from build123d import *

# Parameters (mm, degrees)
SKETCH1_R           = 36
SKETCH1_R_2         = 31.1
BOSS_EXTRUDE1_DEPTH = 15
SKETCH2_R           = 36
BOSS_EXTRUDE2_DEPTH = 5
SKETCH3_R           = 22.5
CUT_EXTRUDE1_DEPTH  = 5
SKETCH4_R           = 5
BOSS_EXTRUDE3_DEPTH = 20
BOSS_EXTRUDE4_DEPTH = 20
SKETCH7_R           = 2.25
CUT_EXTRUDE2_DEPTH  = 78.645922206
SKETCH9_W           = 8.35
SKETCH9_H           = 20
BOSS_EXTRUDE5_DEPTH = 10
FILLET1_R           = 12
SKETCH10_R          = 3
CUT_EXTRUDE3_DEPTH  = 30
CUT_EXTRUDE5_START  = -5
SKETCH10_4_R        = 5.5
SKETCH10_4_R_2      = 3
CUT_EXTRUDE5_DEPTH  = 25
FILLET2_R           = 3
FILLET3_R           = 1


with BuildPart() as part:
    # Sketch1 → Boss-Extrude1 (new body)
    with BuildSketch(Plane.XY):
        Circle(SKETCH1_R)
        Circle(SKETCH1_R_2, mode=Mode.SUBTRACT)
    extrude(amount=BOSS_EXTRUDE1_DEPTH)

    # Sketch2 → Boss-Extrude2 (add)
    with BuildSketch(Plane.XY.offset(15)):
        Circle(SKETCH2_R)
    extrude(amount=BOSS_EXTRUDE2_DEPTH)

    # Sketch3 → Cut-Extrude1 (cut)
    with BuildSketch(Plane.XY.offset(20)):
        Circle(SKETCH3_R)
    extrude(amount=-CUT_EXTRUDE1_DEPTH, mode=Mode.SUBTRACT)

    # Sketch4 → Boss-Extrude3 (add)
    with BuildSketch(Plane(origin=(0, 0, 0), x_dir=(-1, 0, 0), z_dir=(0, 0, -1))):
        with Locations((0, 36.1)):
            Circle(SKETCH4_R)
        with Locations((31.263517077, 18.05)):
            Circle(SKETCH4_R)
        with Locations((31.263517077, -18.05)):
            Circle(SKETCH4_R)
        with Locations((0, -36.1)):
            Circle(SKETCH4_R)
        with Locations((-31.263517077, -18.05)):
            Circle(SKETCH4_R)
        with Locations((-31.263517077, 18.05)):
            Circle(SKETCH4_R)
    extrude(amount=-BOSS_EXTRUDE3_DEPTH)

    # Sketch8 → Boss-Extrude4 (add)
    with BuildSketch(Plane(origin=(0, 0, 0), x_dir=(-1, 0, 0), z_dir=(0, 0, -1))):
        with BuildLine():
            Line((-28.387135314, -22.139795588), (-9.877135314, -54.200056036))
            Line((-9.877135314, -54.200056036), (51.877193071, -18.54617792))
            Line((51.877193071, -18.54617792), (33.367193071, 13.514082528))
            ThreePointArc((33.367193071, 13.514082528), (18, -31.176914536), (-28.387135314, -22.139795588))
        make_face()
    extrude(amount=-BOSS_EXTRUDE4_DEPTH)

    # Sketch7 → Cut-Extrude2 (cut, through all)
    with BuildSketch(Plane(origin=(0, 0, 0), x_dir=(-1, 0, 0), z_dir=(0, 0, -1))):
        with Locations((-31.263517077, 18.05)):
            Circle(SKETCH7_R)
        with Locations((0, 36.1)):
            Circle(SKETCH7_R)
        with Locations((31.263517077, 18.05)):
            Circle(SKETCH7_R)
        with Locations((31.263517077, -18.05)):
            Circle(SKETCH7_R)
        with Locations((0, -36.1)):
            Circle(SKETCH7_R)
        with Locations((-31.263517077, -18.05)):
            Circle(SKETCH7_R)
    extrude(amount=-CUT_EXTRUDE2_DEPTH, mode=Mode.SUBTRACT)

    # Sketch9 → Boss-Extrude5 (add)
    with BuildSketch(Plane(origin=(-21.000028879, -36.373116978, 0), x_dir=(0.8660254037844385, -0.5000000000000004, 0), z_dir=(-0.5000000000000003, -0.8660254037844384, 0))):
        with Locations((-39.828878116, 10)):
            Rectangle(SKETCH9_W, SKETCH9_H)
        with Locations((39.828878116, 10)):
            Rectangle(SKETCH9_W, SKETCH9_H)
    extrude(amount=-BOSS_EXTRUDE5_DEPTH)

    # Fillet1
    # the kernel refuses this fillet: 12 mm, written as the material it adds along each edge
    with BuildSketch(Plane(origin=(-46.877193071, -9.885923882, 20), x_dir=(-0.8660254037844379, 0.500000000000001, 0), z_dir=(0, 0, -1))) as fillet1_piece_1:
        with BuildLine():
            CenterArc((12, 11.431425983), FILLET1_R, 180, 72.29196439)
            Line((0, 11.431425983), (-0.24, 11.431425983))
            Line((-0.24, 11.431425983), (-0.24, 0))
            Line((-0.24, 0), (0, -0.24))
            ThreePointArc((0, -0.24), (4.175, -0.24), (8.277, -0.22862852))
            Line((8.277, -0.22862852), (8.35, 0))
        make_face()
    extrude(amount=20)
    with BuildSketch(Plane(origin=(14.877135314, -45.539801998, 20), x_dir=(0.5000000000000003, 0.8660254037844385, 0), z_dir=(0, 0, -1))) as fillet1_piece_2:
        with BuildLine():
            CenterArc((11.431425983, 12), FILLET1_R, 197.70803561, 72.29196439)
            Line((0, 8.35), (-0.22862852, 8.277))
            ThreePointArc((-0.22862852, 8.277), (-0.24, 4.175), (-0.24, 0))
            Line((-0.24, 0), (0, -0.24))
            Line((0, -0.24), (11.431425983, -0.24))
            Line((11.431425983, -0.24), (11.431425983, 0))
        make_face()
    extrude(amount=20)

    # Sketch10 → Cut-Extrude3 (cut)
    with BuildSketch(Plane(origin=(-21.000028879, -36.373116978, 0), x_dir=(0.8660254037844385, -0.5000000000000004, 0), z_dir=(-0.5000000000000003, -0.8660254037844384, 0))):
        with Locations((37.503878116, 10)):
            Circle(SKETCH10_R)
        with Locations((-37.503878116, 10)):
            Circle(SKETCH10_R)
    extrude(amount=-CUT_EXTRUDE3_DEPTH, mode=Mode.SUBTRACT)

    # Sketch10<4> → Cut-Extrude5 (cut)
    # profile 1 of 2: a face of its own
    with BuildSketch(Plane(origin=(-21.000028879, -36.373116978, 0), x_dir=(0.8660254037844385, -0.5000000000000004, 0), z_dir=(-0.5000000000000003, -0.8660254037844384, 0)).offset(CUT_EXTRUDE5_START)):
        with Locations((37.503878116, 10)):
            Circle(SKETCH10_4_R)
        with Locations((37.503878116, 10)):
            Circle(SKETCH10_4_R_2, mode=Mode.SUBTRACT)
    # profile 2 of 2: a face of its own
    with BuildSketch(Plane(origin=(-21.000028879, -36.373116978, 0), x_dir=(0.8660254037844385, -0.5000000000000004, 0), z_dir=(-0.5000000000000003, -0.8660254037844384, 0)).offset(CUT_EXTRUDE5_START)):
        with Locations(Location((-37.503878116, 10, 0), (0, 0, 289.655481315))):
            Circle(SKETCH10_4_R)
        with Locations((-37.503878116, 10)):
            Circle(SKETCH10_4_R_2, mode=Mode.SUBTRACT)
    extrude(amount=-CUT_EXTRUDE5_DEPTH, mode=Mode.SUBTRACT)

    # Fillet2
    fillet2_edges = [part.edges().sort_by_distance(p)[0] for p in [
        (-56.608505192, -10.041050901, 0),
        (-56.608505192, -10.041050901, 20),
        (19.608447435, -54.044929017, 0),
        (19.608447435, -54.044929017, 20),
    ]]
    fillet(fillet2_edges, radius=FILLET2_R)

    # Fillet3
    fillet3_edges = [part.edges().sort_by_distance(p)[0] for p in [
        (-52.581487065, -12.366050901, 15.179527005),
        (9.21614259, -48.044929017, 10),
    ]]
    fillet(fillet3_edges, radius=FILLET3_R)


solid = part.part
Could you check a few things on this model? Use its own coordinates, in mm. A direction names the side the tool comes from. Coordinates: 2 decimals unless noted, no trailing zeros. Loops run counter-clockwise (first coordinate to the right, second up) from the corner with the lowest first, then second, coordinate; pieces in that order, holes last.
1. Imagine slicing it at C-C (z = 1.5). Please give me the cut outline in (x, y).
2. Imagine slicing it at D-D (x = -19.5). Please give me the cut outline in (y, z), and give its area (3 significant figures).
3. We'd pull the mould along Y, two halves only. Please class faces 4 (the face through (-56.644, -10.102, 9.902)), 5 (the face through (19.57, -54.11, 9.9)), 6 (the face through (0.29, 38.33, 9.86)): released by +Y, released by -Y, zero draft, split by the parting line, or undercut.
4. For faces 1 (the face through (-36.453, 8.17, 9.86)), 2 (the face through (-35.55, 6.67, 10.62)), 3 (the face through (19.23, -52.9, 0.86)), which set-ups out of +Z, -Z, +X, -X, +Y, -Y let a thin tool reach every point of the face, with its end or its side?
5. Imagine slicing it at A-A (x = 0). Please give me the cut outline in (y, z).
6. Imagine slicing it at B-B (y = 9). Please give me the cut outline in (x, z), and give its area (3 significant figures).
7. I need wall thicknesses on L1, parallel to Y at x = 10.5, z = 13; L2, parallel to Y at x = 0, z = 6.75; L3, parallel to Y at x = 21.5, z = 7.75. Which ranges of each line are inside material? Lowest first, please.
8. For P1, Ø7, axis at x = 31.26, y = 18.05, coming from the -Z side; P2, Ø12, axis at x = -13.5, z = 3.5, coming from the +Y side; P3, Ø4, axis at x = 26, z = 5.5, coming from the -Y side; P4, Ø2, axis at x = -31, z = 4.5, coming from the -Y side, each with a flat end and sliding along its axis, tell me the tip position at first contact or that it passes through.
Computed values:
1. outline: (-58.76, -14.57) - (16.76, -58.17) - (21.83, -49.4) arc R12 cw to (20.59, -35.64) - (28.39, -22.14) arc R5 ccw (long way) to (33.37, -13.51) arc R36 ccw to (33.37, 13.51) arc R5 ccw (long way) to (28.39, 22.14) arc R36 ccw to (4.98, 35.65) arc R5 ccw (long way) to (-4.98, 35.65) arc R36 ccw to (-28.39, 22.14) arc R5 ccw (long way) to (-33.37, 13.51) - (-41.16, 0.01) arc R12 cw to (-53.69, -5.79) - close; hole circle Ø4.5 at (-31.26, -18.05); hole circle Ø4.5 at (-31.26, 18.05); hole circle Ø62.2 at (0, 0); hole circle Ø4.5 at (0, -36.1); hole circle Ø4.5 at (0, 36.1); hole circle Ø4.5 at (31.26, -18.05); hole circle Ø4.5 at (31.26, 18.05)
2. outline: (-37.24, 0) - (-24.23, 0) - (-24.23, 15) - (-11.22, 15) - (-11.22, 20) - (-37.24, 20) - close; (11.22, 15) - (24.23, 15) - (24.23, 0) - (30.26, 0) - (30.26, 20) - (11.22, 20) - close
2. area: 511 mm2
3. face 4: released by +Y
3. face 5: released by -Y
3. face 6: undercut
4. face 1: +Z, -Z, -X
4. face 2: -X
4. face 3: -Z, +X, -Y
5. outline: (-48.5, 0) - (-38.35, 0) - (-38.35, 20) - (-48.5, 20) - close; (-33.85, 0) - (-31.1, 0) - (-31.1, 15) - (-22.5, 15) - (-22.5, 20) - (-33.85, 20) - close; (22.5, 15) - (31.1, 15) - (31.1, 0) - (33.85, 0) - (33.85, 20) - (22.5, 20) - close; (38.35, 0) - (41.1, 0) - (41.1, 20) - (38.35, 20) - close
6. outline: (-35.97, 0) - (-29.77, 0) - (-29.77, 15) - (-20.62, 15) - (-20.62, 20) - (-35.97, 20) - close; (20.62, 15) - (29.77, 15) - (29.77, 0) - (34.86, 0) - (34.86, 20) - (20.62, 20) - close
6. area: 317 mm2
7. L1: y = -54.56 to -48.55, -47.6 to -29.27, 29.27 to 34.43
7. L2: y = -48.5 to -38.35, -33.85 to -31.1, 31.1 to 33.85, 38.35 to 41.1
7. L3: y = -50.77 to -48.99, -27.73 to -22.47, 22.47 to 28.87
8. P1: stops at z = 0
8. P2: stops at y = 35.21
8. P3: stops at y = -29.53
8. P4: stops at y = -31.18
